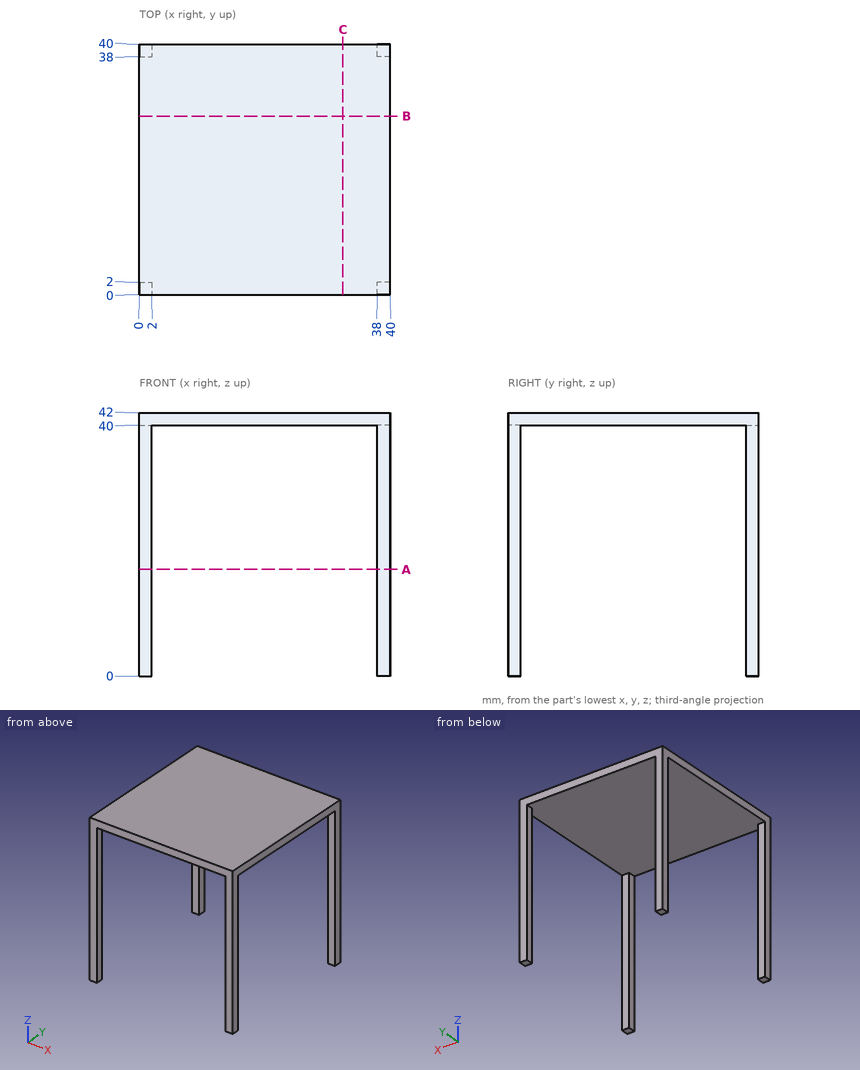
Could you check a few things on this drawing? It's one solid part, dimensions in mm from its lowest x, y, z. Coordinates: 2 decimals unless noted, no trailing zeros. Write each loop counter-clockwise with the first axis right and the second up, starting at its lowest first coordinate (ties: lowest second). Pieces come first, ordered by that corner, then holes. Notation, with made-up numbers: M 64,1.25 L 72,1.25 A9 cw 72,15.25 Z; hole C -38,54 d7. An arc over 180 degrees is marked long. One line per question, with ' | ' between items.
1) Imagine slicing it at A-A, the plane z = 17. Write out the boundary of the cut face in (x, y), and give its area (3 significant figures).
Checks:
outline: M 0,0 L 2,0 L 2,2 L 0,2 Z; M 0,38 L 2,38 L 2,40 L 0,40 Z; M 38,0 L 40,0 L 40,2 L 38,2 Z; M 38,38 L 40,38 L 40,40 L 38,40 Z | area: 16.0 mm²
2) I need wall thicknesses on probe 1 along Z at (x, y) = (28, 20). Which ranges of the line are inside material? Lowest first, please. Write a range as [from, to].
Checks:
probe 1: [40, 42]
3) For pin 1 Ø5 at (x, y) = (22, 23.5) entering from -Z, with a flat end and sliding along its axis, tell me the tip position at first contact or that it passes through.
Checks:
pin 1: z = 40
4) Imagine slicing it at B-B, the plane y = 28.5. Write out the boundary of the cut face in (x, z).
Checks:
outline: M 0,40 L 40,40 L 40,42 L 0,42 Z
